```python
from build123d import *

# Parameters (mm, degrees)
SKETCH1_W           = 10.5
SKETCH1_H           = 5.5
BOSS_EXTRUDE1_DEPTH = 4.5
SKETCH2_R           = 0.6
BOSS_EXTRUDE2_DEPTH = 6


with BuildPart() as part:
    # Sketch1 → Boss-Extrude1 (new body)
    with BuildSketch(Plane.XY):
        with Locations((5.25, 2.75)):
            Rectangle(SKETCH1_W, SKETCH1_H)
    extrude(amount=BOSS_EXTRUDE1_DEPTH)

    # Sketch2 → Boss-Extrude2 (add)
    with BuildSketch(Plane(origin=(0, 0, 0), x_dir=(-1, 0, 0), z_dir=(0, 0, -1))):
        with Locations((-9.25, 3.75)):
            Circle(SKETCH2_R)
        with Locations((-9.25, 1.75)):
            Circle(SKETCH2_R)
        with Locations((-5.25, 1.75)):
            Circle(SKETCH2_R)
        with Locations((-7.25, 1.75)):
            Circle(SKETCH2_R)
        with Locations((-7.25, 3.75)):
            Circle(SKETCH2_R)
        with Locations((-5.25, 3.75)):
            Circle(SKETCH2_R)
        with Locations((-3.25, 3.75)):
            Circle(SKETCH2_R)
        with Locations((-1.25, 3.75)):
            Circle(SKETCH2_R)
        with Locations((-1.25, 1.75)):
            Circle(SKETCH2_R)
        with Locations((-3.25, 1.75)):
            Circle(SKETCH2_R)
    extrude(amount=BOSS_EXTRUDE2_DEPTH)


solid = part.part
```
CAD build for the part. Positions are in the model's coordinates, mm. A direction names the side the tool comes from. Round coordinates to 2 decimals unless told otherwise and drop trailing zeros. Loops run counter-clockwise (first coordinate to the right, second up) from the corner with the lowest first, then second, coordinate; pieces in that order, holes last. Notation, with made-up numbers: M 51.25,-24.75 L 79.25,-24.75 A30 cw 79.25,5.25 Z; hole C 56.5,63.5 d9. An arc over 180 degrees is marked long. Return JSON: item names as keys, results as strings. Group by question number.
(1) Wall check: probe 1 along X at (y, z) = (3.4, -0.75); probe 2 along Y at (x, z) = (1.25, -2.75); probe 3 along Z at (x, y) = (5.25, 0.35). Give the ranges that are in metal, low to high. Write a range as [from, to].
(2) Saw through at B-B, the plane z = -0.5. Give the number of separate pieces and of enclosed holes in the cut face, and give its area (3 significant figures).
(3) Saw through at C-C, the plane x = 7.25. List the corners of the cut face in (y, z), and give its area (4 significant figures).
(4) Tool access for faces 1 (the cylindrical face through (9.69, 4.16, -2.96)), 2 (the flat face through (3, 2, -6)): list every direction of +Z, -Z, +X, -X, +Y, -Y with a clear straight run to the whole face (end or side of a thin tool).
(5) Drop flat-ended pins along their axis: P1, Ø1, axis at y = 2, z = -1.5, coming from the -X side; P2, Ø2, axis at y = 1, z = -3.5, coming from the +X side; P3, Ø1.5, axis at x = 5, z = -3, coming from the -Y side. Give the stop position or say it passes through.
(6) Saw through at A-A, the plane y = 3.75. List the corners of the cut face in (x, z), and give its area (4 significant figures).
(7) Saw through at D-D, the plane x = 3. List the corners of the cut face in (y, z), and give its area (3 significant figures).
(8) Mould opens along Y. For faces 3 (the flat face through (1, 2, -6)), 4 (the cylindrical face through (3.69, 4.16, -2.96)), 5 (the flat face through (5, 5.5, 2)) say: +Y half, -Y half, draft (parallel to the pull), parting line (faces both ways), or undercut.
Answer list:
{
 "1": {"probe 1": "[0.76, 1.74], [2.76, 3.74], [4.76, 5.74], [6.76, 7.74], [8.76, 9.74]", "probe 2": "[1.15, 2.35], [3.15, 4.35]", "probe 3": "[0, 4.5]"},
 "2": {"separate pieces": "10", "enclosed holes": "0", "area": "11.3 mm2"},
 "3": {"outline": "M 0,0 L 1.15,0 L 1.15,-6 L 2.35,-6 L 2.35,0 L 3.15,0 L 3.15,-6 L 4.35,-6 L 4.35,0 L 5.5,0 L 5.5,4.5 L 0,4.5 Z", "area": "39.15 mm2"},
 "4": {"face 1": "-Z", "face 2": "-Z, +X, -X, +Y, -Y"},
 "5": {"P1": "x = 0.65", "P2": "x = 9.85", "P3": "y = 1.15"},
 "6": {"outline": "M 0,0 L 0.65,0 L 0.65,-6 L 1.85,-6 L 1.85,0 L 2.65,0 L 2.65,-6 L 3.85,-6 L 3.85,0 L 4.65,0 L 4.65,-6 L 5.85,-6 L 5.85,0 L 6.65,0 L 6.65,-6 L 7.85,-6 L 7.85,0 L 8.65,0 L 8.65,-6 L 9.85,-6 L 9.85,0 L 10.5,0 L 10.5,4.5 L 0,4.5 Z", "area": "83.25 mm2"},
 "7": {"outline": "M 0,0 L 1.2,0 L 1.2,-6 L 2.3,-6 L 2.3,0 L 3.2,0 L 3.2,-6 L 4.3,-6 L 4.3,0 L 5.5,0 L 5.5,4.5 L 0,4.5 Z", "area": "37.8 mm2"},
 "8": {"face 3": "draft", "face 4": "undercut", "face 5": "+Y half"}
}
